Geometry: final body of the model. Coordinates: model frame, mm. Face numbers are marked on the shaded views. Round coordinates to 2 decimals unless told otherwise and drop trailing zeros. Order: outer loops, then holes, each group sorted by start corner. A loop starts at its lowest first (then second) coordinate and runs counter-clockwise, first axis right, second up. Notation, with made-up numbers: M 50.5,80 L 54.5,80 A15 ccw 54.5,106 Z; hole C -40,43.5 d1. An arc over 180 degrees is marked long. Return JSON: item names as keys, results as strings. Group by question number.
Q1. Cut plane B-B on y = 0. Output: boundary loops of the cut face in (x, z) (3 decimals).
Q2. Cut plane D-D on z = -7.5. Output: boundary loops of the cut face in (x, y).
Q3. Mould query, pull axis Y, two halves, no side actions, for the marked faces 1, 2 and 3. Classes: released by +Y, released by -Y, zero draft, split by the parting line, or undercut.
Q4. Cut plane C-C on z = 1. Output: boundary loops of the cut face in (x, y), and give its area (3 significant figures).
Q5. Contact query for flat-ended pins moving along their axis: pin 1 (3.5 mm diameter, centred on x = -26, y = 16, fed in from -Z); pin 2 (6 mm diameter, centred on y = 29.5, z = 0, fed in from +X); pin 3 (2 mm diameter, centred on x = 21.5, z = -3, fed in from +Y). Output: stop coordinate, or through.
Q6. Ray query, probe 1 along Y at (x, z) = (-1, -4); probe 2 along Y at (x, z) = (-0.5, -3.5); probe 3 along Z at (x, y) = (-4.5, -12). Return the intervals inside material, ascending.
Q7. Cut plane A-A on x = 0. Output: boundary loops of the cut face in (y, z) (3 decimals), and give its area (3 significant figures).
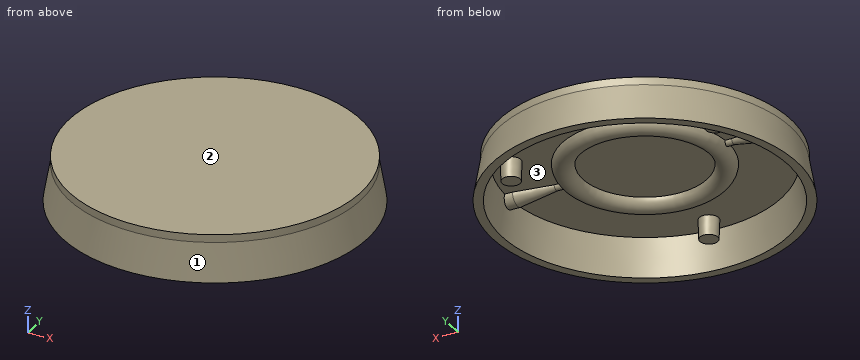
```python
from build123d import *

# Parameters (mm, degrees)
F3_R             = 37.5
F4_DEPTH         = 2
F7_R             = 2.5
F8_DEPTH         = 5
F8_TAPER         = 2
F12_COPIES_COUNT = 2
F14_COPIES_COUNT = 2


# Not quite as in the source:
# - a pattern or mirror of a feature is missing from the dataset's text; its kind, count and spacing are read off the source's solid


with BuildPart() as f2:
    # F1 (on Front) → F2 (revolve)
    with BuildSketch(Plane.XZ):
        with BuildLine():
            Line((-16, 0), (-21.33, 0))
            ThreePointArc((-21.33, 0), (-18.665, -2.665), (-16, 0))
        make_face()
    revolve(axis=Axis((0, 0, 18.396249041), (0, 0, 1)))

    # F3 (on face) → F4 (join)
    with BuildSketch(Plane.XY):
        Circle(F3_R)
    extrude(amount=F4_DEPTH)

    # F5 (on Right) → F6 (revolve)
    with BuildSketch(Plane.YZ):
        Polygon((-36.8366060944, -9.6), (-35.1438670796, 0), (-37.5, 0), (-39.1927390148, -9.6), align=None)
    revolve(axis=Axis((0, 0, 18.396249041), (0, 0, 1)))

    # F7 (on face) → F8 (join)
    with BuildSketch(Plane(origin=(0, 0, 0), x_dir=(1, 0, 0), z_dir=(0, 0, -1))):
        with Locations((0, 30.5)):
            Circle(F7_R)
        with Locations((-26.4137748154, -15.25)):
            Circle(F7_R)
        with Locations((26.4137748154, -15.25)):
            Circle(F7_R)
    extrude(amount=F8_DEPTH, taper=F8_TAPER)

    # F11 (on offset) → F12 (join, up to the next surface of F2)
    with BuildSketch(Plane.YZ.offset(33)):
        with BuildLine():
            Line((2.5, 0), (-2.5, 0))
            ThreePointArc((-2.5, 0), (0, -2.5), (2.5, 0))
        make_face()
    f12 = extrude(until=Until.NEXT)

    # F12_copies: F12 ×2 about axis
    f12_copies_axis = Axis((0, 0, 0), (0, 0, 1))
    for i in range(1, F12_COPIES_COUNT):
        add(f12.rotate(f12_copies_axis, i * 360 / F12_COPIES_COUNT))

    # F13 (on offset) → F14 (join, up to the next surface of F2)
    with BuildSketch(Plane.YZ.offset(23)):
        with BuildLine():
            Line((1, 0), (-1, 0))
            ThreePointArc((-1, 0), (0, -1), (1, 0))
        make_face()
    f14 = extrude(until=Until.NEXT, dir=(-1, 0, 0))

    # F14_copies: F14 ×2 about axis
    f14_copies_axis = Axis((0, 0, 0), (0, 0, 1))
    for i in range(1, F14_COPIES_COUNT):
        add(f14.rotate(f14_copies_axis, i * 360 / F14_COPIES_COUNT))

    # F14_face (on face) → F15 section 0
    with BuildSketch(Plane(origin=(23, 0, -0.4244131816), x_dir=(0, 1, 0), z_dir=(1, 0, 0))):
        with BuildLine():
            Line((1, 0.4244131816), (-1, 0.4244131816))
            ThreePointArc((-1, 0.4244131816), (0, -0.5755868184), (1, 0.4244131816))
        make_face()
    # F12_face (on face) → F15 section 1
    with BuildSketch(Plane(origin=(33, 0, -1.0610329539), x_dir=(0, 1, 0), z_dir=(-1, 0, 0))):
        with BuildLine():
            Line((-2.5, -1.0610329539), (2.5, -1.0610329539))
            ThreePointArc((2.5, -1.0610329539), (0, 1.4389670461), (-2.5, -1.0610329539))
        make_face()
    f15 = loft()

    # F15_copies: F15 across plane
    add(f15.mirror(Plane(origin=(0, 0, 0), x_dir=(0, 0, -1), z_dir=(-1, 0, 0))))


solid = f2.part
```
Result sheet:
{
 "1": {"outline": "M -39.193,-9.6 L -36.837,-9.6 L -35.585,-2.5 L -33,-2.5 L -23,-1 L -21.135,-1 A2.665 ccw -16,0 L 16,0 A2.665 ccw 21.135,-1 L 23,-1 L 33,-2.5 L 35.585,-2.5 L 36.837,-9.6 L 39.193,-9.6 L 37.5,0 L 37.5,2 L -37.5,2 L -37.5,0 Z"},
 "2": {"outline": "C 0,0 d77.64; hole C 0,0 d72.93"},
 "3": {"face 1": "split by the parting line", "face 2": "zero draft", "face 3": "undercut"},
 "4": {"outline": "C 0,0 d75", "area": "4,420 mm²"},
 "5": {"pin 1": "stops at z = -5", "pin 2": "stops at x = 26.62", "pin 3": "stops at y = 32.06"},
 "6": {"probe 1": "y = -38.19 to -35.84, -32.64 to -28.36, 35.84 to 38.19", "probe 2": "y = -38.11 to -35.76, -32.82 to -28.18, 35.76 to 38.11", "probe 3": "z = 0 to 2"},
 "7": {"outline": "M -39.193,-9.6 L -36.837,-9.6 L -35.144,0 L -33,0 L -32.825,-5 L -28.175,-5 L -28,0 L -21.33,0 A2.665 ccw -16,0 L 16,0 A2.665 ccw 21.33,0 L 35.144,0 L 36.837,-9.6 L 39.193,-9.6 L 37.5,0 L 37.5,2 L -37.5,2 L -37.5,0 Z", "area": "242 mm²"}
}
